```python
from build123d import *

# Parameters (mm, degrees)
F0_R     = 59.80071
F0_R_2   = 6.809169
F0_R_3   = 24.331807
F1_DEPTH = 12.7


with BuildPart() as f1:
    # F0 (on Front) → F1 (new body, symmetric)
    with BuildSketch(Plane.XZ):
        Circle(F0_R)
        with Locations((-31.582093, -31.582093)):
            Circle(F0_R_2, mode=Mode.SUBTRACT)
        with Locations((0, -44.663824)):
            Circle(F0_R_2, mode=Mode.SUBTRACT)
        with Locations((31.582093, -31.582093)):
            Circle(F0_R_2, mode=Mode.SUBTRACT)
        with Locations((-44.663824, 0)):
            Circle(F0_R_2, mode=Mode.SUBTRACT)
        with Locations((-31.582093, 31.582093)):
            Circle(F0_R_2, mode=Mode.SUBTRACT)
        Circle(F0_R_3, mode=Mode.SUBTRACT)
        with Locations((44.663824, 0)):
            Circle(F0_R_2, mode=Mode.SUBTRACT)
        with Locations((0, 44.663824)):
            Circle(F0_R_2, mode=Mode.SUBTRACT)
        with Locations((31.582093, 31.582093)):
            Circle(F0_R_2, mode=Mode.SUBTRACT)
    extrude(amount=F1_DEPTH, both=True)


solid = f1.part
```
The listing builds one solid part. Answer for the finished solid, in the listing's coordinates (mm). Coordinates: 2 decimals unless noted, no trailing zeros. Loops run counter-clockwise (first coordinate to the right, second up) from the corner with the lowest first, then second, coordinate; pieces in that order, holes last. Notation, with made-up numbers: (26.25, -17) -> (32.25, -17) arc R24 ccw to (32.25, -4) -> close; hole circle Ø2 at (37.25, -16). An arc over 180 degrees is marked (long way). Return JSON: item names as keys, results as strings. Group by question number.
(1) A cutting plane is placed at C-C on z = 34. Write down the section's boundary in (x, y).
(2) A cutting plane is placed at A-A on z = 0. Write down the section's boundary in (x, y), and give its area (3 significant figures).
(3) Given pin 1 Ø1 at (y, z) = (-8.5, -27.5) entering from +X; pin 2 Ø4 at (y, z) = (3.5, -11.5) entering from -X; pin 3 Ø8 at (x, y) = (-6.5, -3.5) entering from +Z, each flat-ended and moving along its own axis, determine where each tip first touches the part or whether it passes through.
(4) A cutting plane is placed at D-D on y = 2. Count the separate pieces of the cut face and the enclosed holes in it, and give its area (3 significant figures).
(5) A cutting plane is placed at B-B on x = 0. Write down the section's boundary in (y, z).
(6) Find the intervals of material crossed by probe 1 along Z at (x, y) = (0, -1); probe 2 along Z at (x, y) = (4.5, 5.5); probe 3 along X at (y, z) = (9.5, 31.5), in increasing order. Write a range as from..to.
(7) Determine the mould class of faces 1 (the flat face through (26, -12.7, 1)), 2 (the cylindrical face through (-1.476, 0.178, 38.017)), 3 (the cylindrical face through (57.04, -0.18, 17.96)) for opening direction X: released by +X, released by -X, zero draft, split by the parting line, or undercut.
The answers:
{
 "1": {"outline": "(-49.19, -12.7) -> (-37.95, -12.7) -> (-37.95, 12.7) -> (-49.19, 12.7) -> close; (-25.22, -12.7) -> (25.22, -12.7) -> (25.22, 12.7) -> (-25.22, 12.7) -> close; (37.95, -12.7) -> (49.19, -12.7) -> (49.19, 12.7) -> (37.95, 12.7) -> close"},
 "2": {"outline": "(-59.8, -12.7) -> (-51.47, -12.7) -> (-51.47, 12.7) -> (-59.8, 12.7) -> close; (-37.85, -12.7) -> (-24.33, -12.7) -> (-24.33, 12.7) -> (-37.85, 12.7) -> close; (24.33, -12.7) -> (37.85, -12.7) -> (37.85, 12.7) -> (24.33, 12.7) -> close; (51.47, -12.7) -> (59.8, -12.7) -> (59.8, 12.7) -> (51.47, 12.7) -> close", "area": "1,110 mm^2"},
 "3": {"pin 1": "stops at x = 53.36", "pin 2": "stops at x = -59.04", "pin 3": "stops at z = 59.75"},
 "4": {"separate pieces": "1", "enclosed holes": "9", "area": "8,210 mm^2"},
 "5": {"outline": "(-12.7, -59.8) -> (12.7, -59.8) -> (12.7, -51.47) -> (-12.7, -51.47) -> close; (-12.7, -37.85) -> (12.7, -37.85) -> (12.7, -24.33) -> (-12.7, -24.33) -> close; (-12.7, 24.33) -> (12.7, 24.33) -> (12.7, 37.85) -> (-12.7, 37.85) -> close; (-12.7, 51.47) -> (12.7, 51.47) -> (12.7, 59.8) -> (-12.7, 59.8) -> close"},
 "6": {"probe 1": "z = -59.8..-51.47, -37.85..-24.33, 24.33..37.85, 51.47..59.8", "probe 2": "z = -59.63..-49.77, -39.55..-23.91, 23.91..39.55, 49.77..59.63", "probe 3": "x = -50.83..-38.39, -24.77..24.77, 38.39..50.83"},
 "7": {"face 1": "zero draft", "face 2": "undercut", "face 3": "split by the parting line"}
}
